The listing builds one solid part. Answer for the finished solid, in the listing's coordinates (mm). Face numbers are marked on the shaded views. A direction names the side the tool comes from. Give positions to 0.01 mm unless a question says otherwise; leave off trailing zeros. Loops run counter-clockwise (first coordinate to the right, second up) from the corner with the lowest first, then second, coordinate; pieces in that order, holes last. Notation, with made-up numbers: M 5.25,80.5 L 51.25,80.5 A16 cw 51.25,108.5 Z; hole C 9,-2.75 d1. An arc over 180 degrees is marked long. One line per item, written item: value. Start each with the question number.
Q1. Consider L1, parallel to X at y = 8, z = 5.75; L2, parallel to Z at x = 5, y = 14.5. Determine where each line is inside the solid, lowest interval first.
Q2. The mould has two halves that part along Y. Classify the marked faces 1, 2 and 3: +Y half, -Y half, draft (parallel to the pull), parting line (faces both ways), or undercut.
Q3. A flat-ended cylindrical pin translates along its axis: pin 1 (1.5 mm diameter, centred on x = 6.5, y = 13.5, fed in from +Z). Find the tip coordinate at first contact, or state that the pin passes through.
Q4. A cutting plane is placed at B-B, the plane y = 14. Determine the outline of the cut face in (x, z), and give its area (3 significant figures).
Q5. For the marked faces 4 and 5, determine the directions among +Z, -Z, +X, -X, +Y, -Y from which every point of the face is accessible in a straight line to the end or side of a thin tool.
Q6. A cutting plane is placed at A-A, the plane z = 11. Determine the outline of the cut face in (x, y), and give its area (3 significant figures).
from build123d import *

# Parameters (mm, degrees)
BOX003_W     = 4.9
BOX003_H     = 12.4
BOX003_DEPTH = 25
BOX002_W     = 4.9
BOX002_H     = 12.4
BOX002_DEPTH = 25
BOX001_W     = 4.9
BOX001_H     = 12.4
BOX001_DEPTH = 25
BOX_W        = 52
BOX_H        = 20
BOX_DEPTH    = 15


with BuildPart() as box003:
    # Box003 → Box003 (new body)
    with BuildSketch(Plane(origin=(23, 4, 2), x_dir=(1, 0, 0), z_dir=(0, 0, 1))):
        with Locations((2.45, 6.2)):
            Rectangle(BOX003_W, BOX003_H)
    extrude(amount=BOX003_DEPTH)


with BuildPart() as box002:
    # Box002 → Box002 (new body)
    with BuildSketch(Plane(origin=(43, 4, 2), x_dir=(1, 0, 0), z_dir=(0, 0, 1))):
        with Locations((2.45, 6.2)):
            Rectangle(BOX002_W, BOX002_H)
    extrude(amount=BOX002_DEPTH)


with BuildPart() as box001:
    # Box001 → Box001 (new body)
    with BuildSketch(Plane(origin=(4, 4, 2), x_dir=(1, 0, 0), z_dir=(0, 0, 1))):
        with Locations((2.45, 6.2)):
            Rectangle(BOX001_W, BOX001_H)
    extrude(amount=BOX001_DEPTH)


with BuildPart() as cut002:
    # Box → Box (new body)
    with BuildSketch(Plane.XY):
        with Locations((26, 10)):
            Rectangle(BOX_W, BOX_H)
    extrude(amount=BOX_DEPTH)

    # Cut: cut Box001
    add(box001.part, mode=Mode.SUBTRACT)

    # Cut001: cut Box002
    add(box002.part, mode=Mode.SUBTRACT)

    # Cut002: cut Box003
    add(box003.part, mode=Mode.SUBTRACT)


solid = cut002.part
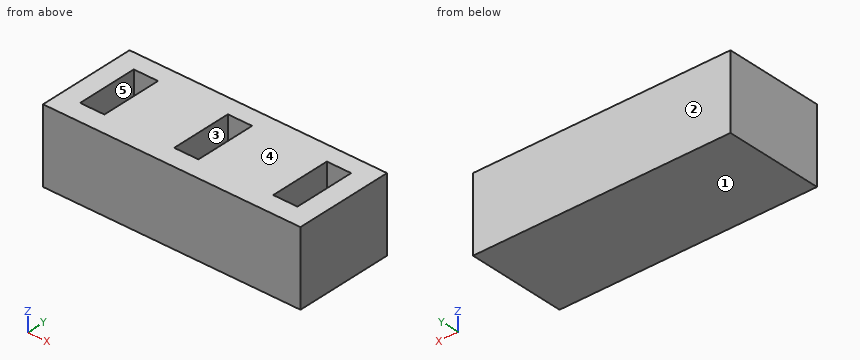
Answer block:
1. L1: 0 to 4, 8.9 to 23, 27.9 to 43, 47.9 to 52
1. L2: 0 to 2
2. face 1: draft
2. face 2: +Y half
2. face 3: undercut
3. pin 1: z = 2
4. outline: M 0,0 L 52,0 L 52,15 L 47.9,15 L 47.9,2 L 43,2 L 43,15 L 27.9,15 L 27.9,2 L 23,2 L 23,15 L 8.9,15 L 8.9,2 L 4,2 L 4,15 L 0,15 Z
4. area: 589 mm^2
5. face 4: +Z, +X, -X, +Y, -Y
5. face 5: +Z
6. outline: M 0,0 L 52,0 L 52,20 L 0,20 Z; hole M 4,4 L 8.9,4 L 8.9,16.4 L 4,16.4 Z; hole M 23,4 L 27.9,4 L 27.9,16.4 L 23,16.4 Z; hole M 43,4 L 47.9,4 L 47.9,16.4 L 43,16.4 Z
6. area: 858 mm^2
